For this review, take the finished solid that the model builds, in its own axes (mm). A direction names the side the tool comes from. Round coordinates to 2 decimals unless told otherwise and drop trailing zeros. Write each loop counter-clockwise with the first axis right and the second up, starting at its lowest first coordinate (ties: lowest second). Pieces come first, ordered by that corner, then holes. Notation, with made-up numbers: (23.5, 63) -> (30.5, 63) arc R22 ccw to (30.5, 70) -> close; hole circle Ø7 at (56.5, 35). An arc over 180 degrees is marked (long way). Write each question's results on one line, items separated by ' | '. Start each with the question number.
Item 1: Add section A-A (x = 19). State the section outline as (y, z) points.
Item 2: To check wall thickness, follow line 1 along Z through (x, y) = (5, 88); line 2 along X through (y, z) = (58.5, -6); line 3 along X through (y, z) = (143.5, -25). State the ranges of each line that lie inside material, in increasing order.
Item 3: Add section D-D (y = 122.25). State the section outline as (x, z) points.
Item 4: Clearance check with flat-ended pins moving along their axes: pin 1 (12 mm diameter, centred on x = 122, y = 35, fed in from +Z); pin 2 (5 mm diameter, centred on x = 60, y = 75, fed in from -Z). State where each tip first meets the part, or that it passes through.
Item 5: Add section B-B (y = 40). State the section outline as (x, z) points, plus the area to 3 significant figures.
Item 6: Add section C-C (x = 167). State the section outline as (y, z) points, plus the area to 3 significant figures.
Item 7: Tool access review of faces 3 (the cylindrical face through (4.93, 88.253, -25.216)), 4 (the flat face through (220, 74, -22)), 5 (the cylindrical face through (44.304, 145.07, -32.436)), 6 (the flat face through (118, 146, -25)): name each direction out of +Z, -Z, +X, -X, +Y, -Y from which nothing blocks a thin tool from reaching the whole face with its end or side.
Item 8: The part is to be moulded in two halves that separate along Z. For faces 1 (the flat face through (5, 115, -5)), 2 (the flat face through (5, 76, -42)), say which applies: +Z half, -Z half, draft (parallel to the pull), parting line (faces both ways), or undercut.
from build123d import *

# Parameters (mm, degrees)
SKETCH1_W           = 230
SKETCH1_H           = 50
BOSS_EXTRUDE1_DEPTH = 150
SKETCH2_W           = 210
SKETCH2_H           = 130
CUT_EXTRUDE1_DEPTH  = 44
SKETCH3_R           = 6.125
CUT_EXTRUDE2_DEPTH  = 4
SKETCH4_R           = 6.125
CUT_EXTRUDE4_DEPTH  = 4
SKETCH5_R           = 6.125
CUT_EXTRUDE5_DEPTH  = 4
SKETCH7_R           = 2
CUT_EXTRUDE7_DEPTH  = 47
SKETCH8_R           = 2
CUT_EXTRUDE8_DEPTH  = 147
CUT_EXTRUDE9_REACH  = 52
SKETCH10_R          = 2
SKETCH10_R_2        = 4.75
SKETCH10_W          = 1.5
SKETCH10_H          = 30
SKETCH11_R          = 7.5
CUT_EXTRUDE10_DEPTH = 151
CUT_EXTRUDE12_REACH = 232
SKETCH14_R          = 0.6
SKETCH15_W          = 5
SKETCH15_H          = 80
CUT_EXTRUDE13_DEPTH = 10
SKETCH16_R          = 2
CUT_EXTRUDE14_DEPTH = 231
CUT_EXTRUDE15_DEPTH = 231


with BuildPart() as part:
    # Sketch1 → Boss-Extrude1 (new body)
    with BuildSketch(Plane(origin=(0, 0, 0), x_dir=(1, 0, 0), z_dir=(0, 1, 0))):
        with Locations((115, 25)):
            Rectangle(SKETCH1_W, SKETCH1_H)
    extrude(amount=BOSS_EXTRUDE1_DEPTH)

    # Sketch2 → Cut-Extrude1 (cut)
    with BuildSketch(Plane.XY):
        with Locations((115, 75)):
            Rectangle(SKETCH2_W, SKETCH2_H)
    extrude(amount=-CUT_EXTRUDE1_DEPTH, mode=Mode.SUBTRACT)

    # Sketch3 → Cut-Extrude2 (cut)
    with BuildSketch(Plane(origin=(0, 150, 0), x_dir=(1, 0, 0), z_dir=(0, 1, 0))):
        with Locations((115, 25)):
            Circle(SKETCH3_R)
    extrude(amount=-CUT_EXTRUDE2_DEPTH, mode=Mode.SUBTRACT)

    # Sketch4 → Cut-Extrude4 (cut)
    with BuildSketch(Plane(origin=(0, 0, 0), x_dir=(1, 0, 0), z_dir=(0, 1, 0))):
        with Locations((115, 25)):
            Circle(SKETCH4_R)
    extrude(amount=CUT_EXTRUDE4_DEPTH, mode=Mode.SUBTRACT)

    # Sketch5 → Cut-Extrude5 (cut)
    with BuildSketch(Plane(origin=(0, 0, -50), x_dir=(-1, 0, 0), z_dir=(0, 0, -1))):
        with Locations((-60, 75)):
            Circle(SKETCH5_R)
    extrude(amount=-CUT_EXTRUDE5_DEPTH, mode=Mode.SUBTRACT)

    # Sketch7 → Cut-Extrude7 (cut, through all)
    with BuildSketch(Plane(origin=(0, 0, -46), x_dir=(-1, 0, 0), z_dir=(0, 0, -1))):
        with Locations((-60, 75)):
            Circle(SKETCH7_R)
    extrude(amount=-CUT_EXTRUDE7_DEPTH, mode=Mode.SUBTRACT)

    # Sketch8 → Cut-Extrude8 (cut, through all)
    with BuildSketch(Plane(origin=(0, 146, 0), x_dir=(1, 0, 0), z_dir=(0, 1, 0))):
        with Locations((115, 25)):
            Circle(SKETCH8_R)
    extrude(amount=-CUT_EXTRUDE8_DEPTH, mode=Mode.SUBTRACT)

    # Sketch10 → Cut-Extrude9 (cut, up to next)
    with BuildSketch(Plane(origin=(0, 0, -50), x_dir=(-1, 0, 0), z_dir=(0, 0, -1)), mode=Mode.PRIVATE) as cut_extrude9_sk1:
        with Locations((-27, 92.5)):
            Circle(SKETCH10_R)
    cut_extrude9_tool1 = extrude(cut_extrude9_sk1.sketch, amount=-CUT_EXTRUDE9_REACH, mode=Mode.PRIVATE) & part.part
    add(cut_extrude9_tool1.solids().sort_by_distance((27, 92.5, -50))[0], mode=Mode.SUBTRACT)
    # Sketch10 → Cut-Extrude9 (cut, up to next)
    with BuildSketch(Plane(origin=(0, 0, -50), x_dir=(-1, 0, 0), z_dir=(0, 0, -1)), mode=Mode.PRIVATE) as cut_extrude9_sk2:
        with Locations((-27, 57.5)):
            Circle(SKETCH10_R)
    cut_extrude9_tool2 = extrude(cut_extrude9_sk2.sketch, amount=-CUT_EXTRUDE9_REACH, mode=Mode.PRIVATE) & part.part
    add(cut_extrude9_tool2.solids().sort_by_distance((27, 57.5, -50))[0], mode=Mode.SUBTRACT)
    # Sketch10 → Cut-Extrude9 (cut, up to next)
    with BuildSketch(Plane(origin=(0, 0, -50), x_dir=(-1, 0, 0), z_dir=(0, 0, -1)), mode=Mode.PRIVATE) as cut_extrude9_sk3:
        with Locations((-19, 75)):
            Circle(SKETCH10_R_2)
    cut_extrude9_tool3 = extrude(cut_extrude9_sk3.sketch, amount=-CUT_EXTRUDE9_REACH, mode=Mode.PRIVATE) & part.part
    add(cut_extrude9_tool3.solids().sort_by_distance((19, 75, -50))[0], mode=Mode.SUBTRACT)
    # Sketch10 → Cut-Extrude9 (cut, up to next)
    with BuildSketch(Plane(origin=(0, 0, -50), x_dir=(-1, 0, 0), z_dir=(0, 0, -1)), mode=Mode.PRIVATE) as cut_extrude9_sk4:
        with Locations((-34.018423534, 75)):
            Rectangle(SKETCH10_W, SKETCH10_H)
    cut_extrude9_tool4 = extrude(cut_extrude9_sk4.sketch, amount=-CUT_EXTRUDE9_REACH, mode=Mode.PRIVATE) & part.part
    add(cut_extrude9_tool4.solids().sort_by_distance((34.018424, 75, -50))[0], mode=Mode.SUBTRACT)

    # Sketch11 → Cut-Extrude10 (cut, through all)
    with BuildSketch(Plane(origin=(0, 150, 0), x_dir=(1, 0, 0), z_dir=(0, 1, 0))):
        with Locations((45.280155496, 25)):
            Circle(SKETCH11_R)
        with Locations((150.781597071, 25)):
            Circle(SKETCH11_R)
        with Locations((206.820659907, 25)):
            Circle(SKETCH11_R)
    extrude(amount=-CUT_EXTRUDE10_DEPTH, mode=Mode.SUBTRACT)

    # Sketch14 → Cut-Extrude12 (cut, up to next)
    with BuildSketch(Plane.ZY, mode=Mode.PRIVATE) as cut_extrude12_sk1:
        with Locations((-33.75, 62)):
            Circle(SKETCH14_R)
    cut_extrude12_tool1 = extrude(cut_extrude12_sk1.sketch, amount=-CUT_EXTRUDE12_REACH, mode=Mode.PRIVATE) & part.part
    add(cut_extrude12_tool1.solids().sort_by_distance((0, 62, -33.75))[0], mode=Mode.SUBTRACT)
    # Sketch14 → Cut-Extrude12 (cut, up to next)
    with BuildSketch(Plane.ZY, mode=Mode.PRIVATE) as cut_extrude12_sk2:
        with Locations((-16.25, 19.5)):
            Circle(SKETCH14_R)
    cut_extrude12_tool2 = extrude(cut_extrude12_sk2.sketch, amount=-CUT_EXTRUDE12_REACH, mode=Mode.PRIVATE) & part.part
    add(cut_extrude12_tool2.solids().sort_by_distance((0, 19.5, -16.25))[0], mode=Mode.SUBTRACT)
    # Sketch14 → Cut-Extrude12 (cut, up to next)
    with BuildSketch(Plane.ZY, mode=Mode.PRIVATE) as cut_extrude12_sk3:
        with Locations((-16.25, 62)):
            Circle(SKETCH14_R)
    cut_extrude12_tool3 = extrude(cut_extrude12_sk3.sketch, amount=-CUT_EXTRUDE12_REACH, mode=Mode.PRIVATE) & part.part
    add(cut_extrude12_tool3.solids().sort_by_distance((0, 62, -16.25))[0], mode=Mode.SUBTRACT)
    # Sketch14 → Cut-Extrude12 (cut, up to next)
    with BuildSketch(Plane.ZY, mode=Mode.PRIVATE) as cut_extrude12_sk4:
        with Locations((-33.75, 19.5)):
            Circle(SKETCH14_R)
    cut_extrude12_tool4 = extrude(cut_extrude12_sk4.sketch, amount=-CUT_EXTRUDE12_REACH, mode=Mode.PRIVATE) & part.part
    add(cut_extrude12_tool4.solids().sort_by_distance((0, 19.5, -33.75))[0], mode=Mode.SUBTRACT)
    # Sketch14 → Cut-Extrude12 (cut, up to next)
    with BuildSketch(Plane.ZY, mode=Mode.PRIVATE) as cut_extrude12_sk5:
        with Locations((-33.75, 130.5)):
            Circle(SKETCH14_R)
    cut_extrude12_tool5 = extrude(cut_extrude12_sk5.sketch, amount=-CUT_EXTRUDE12_REACH, mode=Mode.PRIVATE) & part.part
    add(cut_extrude12_tool5.solids().sort_by_distance((0, 130.5, -33.75))[0], mode=Mode.SUBTRACT)
    # Sketch14 → Cut-Extrude12 (cut, up to next)
    with BuildSketch(Plane.ZY, mode=Mode.PRIVATE) as cut_extrude12_sk6:
        with Locations((-16.25, 88)):
            Circle(SKETCH14_R)
    cut_extrude12_tool6 = extrude(cut_extrude12_sk6.sketch, amount=-CUT_EXTRUDE12_REACH, mode=Mode.PRIVATE) & part.part
    add(cut_extrude12_tool6.solids().sort_by_distance((0, 88, -16.25))[0], mode=Mode.SUBTRACT)
    # Sketch14 → Cut-Extrude12 (cut, up to next)
    with BuildSketch(Plane.ZY, mode=Mode.PRIVATE) as cut_extrude12_sk7:
        with Locations((-16.25, 130.5)):
            Circle(SKETCH14_R)
    cut_extrude12_tool7 = extrude(cut_extrude12_sk7.sketch, amount=-CUT_EXTRUDE12_REACH, mode=Mode.PRIVATE) & part.part
    add(cut_extrude12_tool7.solids().sort_by_distance((0, 130.5, -16.25))[0], mode=Mode.SUBTRACT)
    # Sketch14 → Cut-Extrude12 (cut, up to next)
    with BuildSketch(Plane.ZY, mode=Mode.PRIVATE) as cut_extrude12_sk8:
        with Locations((-33.75, 88)):
            Circle(SKETCH14_R)
    cut_extrude12_tool8 = extrude(cut_extrude12_sk8.sketch, amount=-CUT_EXTRUDE12_REACH, mode=Mode.PRIVATE) & part.part
    add(cut_extrude12_tool8.solids().sort_by_distance((0, 88, -33.75))[0], mode=Mode.SUBTRACT)
    # Sketch14 → Cut-Extrude12 (cut, up to next)
    with BuildSketch(Plane.ZY, mode=Mode.PRIVATE) as cut_extrude12_sk9:
        with BuildLine():
            Line((-35.25, 44.99795855), (-35.25, 36.50204145))
            ThreePointArc((-35.25, 36.50204145), (-35.159960979, 35.772571025), (-34.895248599, 35.086887802))
            Line((-34.895248599, 35.086887802), (-32.483314774, 30.578427125))
            ThreePointArc((-32.483314774, 30.578427125), (-25, 19.75), (-17.516685226, 30.578427125))
            Line((-17.516685226, 30.578427125), (-15.104751401, 35.086887802))
            ThreePointArc((-15.104751401, 35.086887802), (-14.840039021, 35.772571025), (-14.75, 36.50204145))
            Line((-14.75, 36.50204145), (-14.75, 44.99795855))
            ThreePointArc((-14.75, 44.99795855), (-14.840039021, 45.727428975), (-15.104751401, 46.413112198))
            Line((-15.104751401, 46.413112198), (-17.516685226, 50.921572875))
            ThreePointArc((-17.516685226, 50.921572875), (-25, 61.75), (-32.483314774, 50.921572875))
            Line((-32.483314774, 50.921572875), (-34.895248599, 46.413112198))
            ThreePointArc((-34.895248599, 46.413112198), (-35.159960979, 45.727428975), (-35.25, 44.99795855))
        make_face()
    cut_extrude12_tool9 = extrude(cut_extrude12_sk9.sketch, amount=-CUT_EXTRUDE12_REACH, mode=Mode.PRIVATE) & part.part
    add(cut_extrude12_tool9.solids().sort_by_distance((0, 40.75, -25))[0], mode=Mode.SUBTRACT)
    # Sketch14 → Cut-Extrude12 (cut, up to next)
    with BuildSketch(Plane.ZY, mode=Mode.PRIVATE) as cut_extrude12_sk10:
        with BuildLine():
            Line((-34.895248599, 103.586887802), (-32.483314774, 99.078427125))
            ThreePointArc((-32.483314774, 99.078427125), (-25, 88.25), (-17.516685226, 99.078427125))
            Line((-17.516685226, 99.078427125), (-15.104751401, 103.586887802))
            ThreePointArc((-15.104751401, 103.586887802), (-14.840039021, 104.272571025), (-14.75, 105.00204145))
            Line((-14.75, 105.00204145), (-14.75, 113.49795855))
            ThreePointArc((-14.75, 113.49795855), (-14.840039021, 114.227428975), (-15.104751401, 114.913112198))
            Line((-15.104751401, 114.913112198), (-17.516685226, 119.421572875))
            ThreePointArc((-17.516685226, 119.421572875), (-25, 130.25), (-32.483314774, 119.421572875))
            Line((-32.483314774, 119.421572875), (-34.895248599, 114.913112198))
            ThreePointArc((-34.895248599, 114.913112198), (-35.159960979, 114.227428975), (-35.25, 113.49795855))
            Line((-35.25, 113.49795855), (-35.25, 105.00204145))
            ThreePointArc((-35.25, 105.00204145), (-35.159960979, 104.272571025), (-34.895248599, 103.586887802))
        make_face()
    cut_extrude12_tool10 = extrude(cut_extrude12_sk10.sketch, amount=-CUT_EXTRUDE12_REACH, mode=Mode.PRIVATE) & part.part
    add(cut_extrude12_tool10.solids().sort_by_distance((0, 109.25, -25))[0], mode=Mode.SUBTRACT)

    # Sketch15 → Cut-Extrude13 (cut)
    with BuildSketch(Plane.XY):
        with Locations((5, 75)):
            Rectangle(SKETCH15_W, SKETCH15_H)
    cut_extrude13 = extrude(amount=-CUT_EXTRUDE13_DEPTH, mode=Mode.SUBTRACT)

    # Sketch16 → Cut-Extrude14 (cut, through all)
    with BuildSketch(Plane.ZY):
        with Locations((-5, 54.275849875)):
            Circle(SKETCH16_R)
        with Locations((-5, 75)):
            Circle(SKETCH16_R)
        with Locations((-5, 95.724150125)):
            Circle(SKETCH16_R)
    extrude(amount=-CUT_EXTRUDE14_DEPTH, mode=Mode.SUBTRACT)

    # Sketch17 → Cut-Extrude15 (cut, through all)
    with BuildSketch(Plane.ZY):
        Polygon((-38, 25), (-37.940213387, 75), (-38, 125), (-42, 125), (-42, 25), align=None)
    extrude(amount=-CUT_EXTRUDE15_DEPTH, mode=Mode.SUBTRACT)

    # Mirror1: Cut-Extrude13 across plane
    add(cut_extrude13.mirror(Plane(origin=(115, 0, 0), x_dir=(0, 0, 1), z_dir=(1, 0, 0))), mode=Mode.SUBTRACT)


solid = part.part
Responses:
1) outline: (0, -50) -> (70.25, -50) -> (70.25, -44) -> (10, -44) -> (10, 0) -> (0, 0) -> close; (79.75, -50) -> (150, -50) -> (150, 0) -> (140, 0) -> (140, -44) -> (79.75, -44) -> close
2) line 1: z = -50 to -42, -37.96 to -34.35, -33.15 to -16.85, -15.65 to -10 | line 2: x = 0 to 2.5, 7.5 to 10, 220 to 222.5, 227.5 to 230 | line 3: x = 0 to 37.78, 52.78 to 113, 117 to 143.28, 158.28 to 199.32, 214.32 to 230
3) outline: (0, -50) -> (230, -50) -> (230, -42) -> (220, -42) -> (220, -44) -> (10, -44) -> (10, -42) -> (0, -42) -> close; (0, -38) -> (10, -38) -> (10, -33) -> (0, -33) -> close; (0, -17) -> (10, -17) -> (10, 0) -> (0, 0) -> close; (220, -38) -> (230, -38) -> (230, 0) -> (220, 0) -> close
4) pin 1: stops at z = -44 | pin 2: stops at z = -46
5) outline: (0, -50) -> (230, -50) -> (230, -42) -> (220, -42) -> (220, -44) -> (10, -44) -> (10, -42) -> (0, -42) -> close; (0, -37.98) -> (10, -37.98) -> (10, -35.25) -> (0, -35.25) -> close; (0, -14.75) -> (10, -14.75) -> (10, 0) -> (7.5, 0) -> (7.5, -10) -> (2.5, -10) -> (2.5, 0) -> (0, 0) -> close; (220, -37.98) -> (230, -37.98) -> (230, 0) -> (227.5, 0) -> (227.5, -10) -> (222.5, -10) -> (222.5, 0) -> (220, 0) -> close | area: 1,870 mm^2
6) outline: (0, -50) -> (150, -50) -> (150, 0) -> (140, 0) -> (140, -44) -> (10, -44) -> (10, 0) -> (0, 0) -> close | area: 1,780 mm^2
7) face 3: -X | face 4: +Z | face 5: +Y, -Y | face 6: +Y
8) face 1: draft | face 2: undercut
